Build history of the part. All positions in model axes, mm. A direction names the side the tool comes from. Coordinates: 2 decimals unless noted, no trailing zeros. Loops run counter-clockwise (first coordinate to the right, second up) from the corner with the lowest first, then second, coordinate; pieces in that order, holes last.
Item 1: Mould opens along X. For faces 1 (the face through (0, 10, 194)), 2 (the face through (206, 12, 379)), 3 (the face through (417, 10, 194)) say: released by +X, released by -X, zero draft, split by the parting line, or undercut.
Item 2: Cut at A-A (y = 10). List the corners of the cut face in (x, z), and give its area (3 significant figures).
Item 3: Drill centre lines: line 1 along Z through (x, y) = (138, 15); line 2 along X through (y, z) = (10.75, 24); line 3 along Y through (x, z) = (415, 349). Where is each one in solid material? Low to high.
Item 4: Cut at B-B (x = 270.5). List the corners of the cut face in (y, z).
Item 5: 3-axis set-ups, long thin cutter, end or side, ignore diameter. For faces 4 (the face through (3, 12, 194)), 5 (the face through (206, 10, 382)): which of +Z, -Z, +X, -X, +Y, -Y reach the whole face in a straight line?
from build123d import *

# Parameters (mm, degrees)
SKETCH_1_W          = 417
SKETCH_1_H          = 382
EXTRUDE_3_DEPTH     = 20
SKETCH_2_W          = 411
SKETCH_2_H          = 376
CUT_EXTRUDE_1_DEPTH = 17
SKETCH_3_R          = 3
CUT_EXTRUDE_2_DEPTH = 418


with BuildPart() as part:
    # 草圖1 → 填料-伸長3 (new body)
    with BuildSketch(Plane(origin=(0, 0, 0), x_dir=(1, 0, 0), z_dir=(0, 1, 0))):
        with Locations((208.5, -191)):
            Rectangle(SKETCH_1_W, SKETCH_1_H)
    extrude(amount=EXTRUDE_3_DEPTH)

    # 草圖2 → 除料-伸長1 (cut)
    with BuildSketch(Plane(origin=(0, 20, 0), x_dir=(1, 0, 0), z_dir=(0, 1, 0))):
        with Locations((208.5, -191)):
            Rectangle(SKETCH_2_W, SKETCH_2_H)
    extrude(amount=-CUT_EXTRUDE_1_DEPTH, mode=Mode.SUBTRACT)

    # 草圖3 → 除料-伸長2 (cut, through all)
    with BuildSketch(Plane(origin=(417, 0, 0), x_dir=(0, 0, -1), z_dir=(1, 0, 0))):
        with Locations((-33, 10)):
            Circle(SKETCH_3_R)
        with Locations((-349, 10)):
            Circle(SKETCH_3_R)
    extrude(amount=-CUT_EXTRUDE_2_DEPTH, mode=Mode.SUBTRACT)


solid = part.part
Filled sheet:
1. face 1: released by -X
1. face 2: undercut
1. face 3: released by +X
2. outline: (0, 0) - (417, 0) - (417, 30) - (414, 30) - (414, 3) - (3, 3) - (3, 30) - (0, 30) - close; (0, 36) - (3, 36) - (3, 346) - (0, 346) - close; (0, 352) - (3, 352) - (3, 379) - (414, 379) - (414, 352) - (417, 352) - (417, 382) - (0, 382) - close; (414, 36) - (417, 36) - (417, 346) - (414, 346) - close
2. area: 4,690 mm2
3. line 1: z = 0 to 3, 379 to 382
3. line 2: x = 0 to 3, 414 to 417
3. line 3: y = 0 to 7, 13 to 20
4. outline: (0, 0) - (20, 0) - (20, 3) - (3, 3) - (3, 379) - (20, 379) - (20, 382) - (0, 382) - close
5. face 4: +Y
5. face 5: +Z, +X, -X, +Y, -Y
